from build123d import *

# Parameters (mm, degrees)
BASE_FLANGE1_DEPTH      = 70
CUT_EXTRUDE1_DEPTH      = 152.657508881
CUT_EXTRUDE1_DEPTH_BACK = 152.657508881
FILLET1_R               = 12
SKETCH7_R               = 4
SKETCH7_R_2             = 6
SKETCH7_R_3             = 7
CUT_EXTRUDE2_DEPTH      = 150.457314712
SKETCH8_R               = 5
CUT_EXTRUDE3_DEPTH      = 10
FILLET2_R               = 3
BOSS_EXTRUDE1_START     = 5
SKETCH9_R               = 10
SKETCH9_R_2             = 7
BOSS_EXTRUDE1_DEPTH     = 5
FILLET3_R               = 5
FILLET4_R               = 3
FILLET5_R               = 3
FILLET6_R               = 5
FILLET7_R               = 5


# Sheet-metal steps are written as plain solids
with BuildPart() as part:
    # Sketch1 → Base-Flange1 (new, symmetric)
    with BuildSketch(Plane(origin=(0, 0, 0), x_dir=(0, 0, -1), z_dir=(1, 0, 0))):
        with BuildLine():
            Line((-45, 100), (-45, 6))
            ThreePointArc((-45, 6), (-43.242640687, 1.757359313), (-39, 0))
            Line((-39, 0), (39, 0))
            ThreePointArc((39, 0), (43.242640687, 1.757359313), (45, 6))
            Line((45, 6), (45, 100))
            Line((45, 100), (42, 100))
            Line((42, 100), (42, 6))
            ThreePointArc((42, 6), (41.121320344, 3.878679656), (39, 3))
            Line((39, 3), (-39, 3))
            ThreePointArc((-39, 3), (-41.121320344, 3.878679656), (-42, 6))
            Line((-42, 6), (-42, 100))
            Line((-42, 100), (-45, 100))
        make_face()
    extrude(amount=BASE_FLANGE1_DEPTH, both=True)

    # Sketch6 → Cut-Extrude1 (cut, two sides: drawn at the far end of the back side and taken through both)
    with BuildSketch(Plane.XY.offset(45).offset(-CUT_EXTRUDE1_DEPTH_BACK)):
        Polygon((-417.259543972, 6), (-70, 6), (-60, 6), (-60, 70), (60, 100), (60, 6), (70, 6), (417.259543972, 6), (417.259543972, 700.519087943), (-417.259543972, 700.519087943), align=None)
    extrude(amount=CUT_EXTRUDE1_DEPTH + CUT_EXTRUDE1_DEPTH_BACK, mode=Mode.SUBTRACT)

    # Fillet1
    fillet1_edges = [part.edges().sort_by_distance(p)[0] for p in [
        (60, 100, -43.5),
        (60, 100, 43.5),
        (-60, 70, -43.5),
        (-60, 70, 43.5),
    ]]
    fillet(fillet1_edges, radius=FILLET1_R)

    # Sketch7 → Cut-Extrude2 (cut, through all)
    with BuildSketch(Plane.XY.offset(45)):
        with Locations((-48, 60.630683123)):
            Circle(SKETCH7_R)
        with Locations((48, 84.630683123)):
            Circle(SKETCH7_R_2)
        with Locations((-23, 38)):
            Circle(SKETCH7_R_3)
    extrude(amount=-CUT_EXTRUDE2_DEPTH, mode=Mode.SUBTRACT)

    # Sketch8 → Cut-Extrude3 (cut)
    with BuildSketch(Plane.XZ):
        with Locations(Location((7, 0, 0), (0, 0, 270))):
            Circle(SKETCH8_R)
        with Locations(Location((-50, 0, 0), (0, 0, 270))):
            Circle(SKETCH8_R)
        with BuildLine():
            Line((26, 5), (50, 5))
            ThreePointArc((50, 5), (55, 0), (50, -5))
            Line((50, -5), (26, -5))
            ThreePointArc((26, -5), (21, 0), (26, 5))
        make_face()
        with BuildLine():
            Line((-45, 27.5), (-45, 22.5))
            ThreePointArc((-45, 22.5), (-50, 17.5), (-55, 22.5))
            Line((-55, 22.5), (-55, 27.5))
            ThreePointArc((-55, 27.5), (-50, 32.5), (-45, 27.5))
        make_face()
        with BuildLine():
            Line((-45, -22.5), (-45, -27.5))
            ThreePointArc((-45, -27.5), (-50, -32.5), (-55, -27.5))
            Line((-55, -27.5), (-55, -22.5))
            ThreePointArc((-55, -22.5), (-50, -17.5), (-45, -22.5))
        make_face()
    extrude(amount=-CUT_EXTRUDE3_DEPTH, mode=Mode.SUBTRACT)

    # Fillet2
    fillet2_edges = [part.edges().sort_by_distance(p)[0] for p in [
        (-70, 6, -43.5),
        (70, 6, -43.5),
        (-70, 6, 43.5),
        (70, 6, 43.5),
    ]]
    fillet(fillet2_edges, radius=FILLET2_R - 0.0001)  # a hair under: the kernel refuses the full size

    # Sketch9 → Boss-Extrude1 (add)
    with BuildSketch(Plane.XY.offset(45).offset(BOSS_EXTRUDE1_START)):
        with Locations(Location((-23, 38, 0), (0, 0, 180))):
            Circle(SKETCH9_R)
        with Locations((-23, 38)):
            Circle(SKETCH9_R_2, mode=Mode.SUBTRACT)
    boss_extrude1 = extrude(amount=-BOSS_EXTRUDE1_DEPTH)

    # Fillet3
    fillet3_edges = [part.edges().sort_by_distance(p)[0] for p in [
        (-13, 38, 45),
    ]]
    fillet(fillet3_edges, radius=FILLET3_R - 0.0001)  # a hair under: the kernel refuses the full size

    # Fillet4
    fillet4_edges = [part.edges().sort_by_distance(p)[0] for p in [
        (-30, 38, 42),
    ]]
    fillet(fillet4_edges, radius=FILLET4_R)

    # Mirror5: Boss-Extrude1 across plane
    add(boss_extrude1.mirror(Plane.XY))

    # Fillet5
    fillet5_edges = [part.edges().sort_by_distance(p)[0] for p in [
        (-30, 38, -42),
    ]]
    fillet(fillet5_edges, radius=FILLET5_R)

    # Fillet6
    fillet6_edges = [part.edges().sort_by_distance(p)[0] for p in [
        (-13, 38, -45),
    ]]
    fillet(fillet6_edges, radius=FILLET6_R - 0.0001)  # a hair under: the kernel refuses the full size

    # Fillet7
    fillet7_edges = [part.edges().sort_by_distance(p)[0] for p in [
        (60, 6, -43.5),
        (60, 6, 43.5),
        (-60, 6, -43.5),
        (-60, 6, 43.5),
    ]]
    fillet(fillet7_edges, radius=FILLET7_R)


solid = part.part
CAD build for the part. Positions are in the model's coordinates, mm. A direction names the side the tool comes from. Give positions to 0.01 mm unless a question says otherwise; leave off trailing zeros. Write each loop counter-clockwise with the first axis right and the second up, starting at its lowest first coordinate (ties: lowest second). Pieces come first, ordered by that corner, then holes. Notation, with made-up numbers: (25.25, 38) -> (40.25, 38) arc R32 cw to (40.25, 75) -> close; hole circle Ø10 at (59, 7.25). An arc over 180 degrees is marked (long way). Return JSON: item names as keys, results as strings.
Item 1: Band-saw the part on D-D (y = 17). List the corners of the cut face in (x, z).
Answer below:
{"outline": "(-60, -45) -> (60, -45) -> (60, -42) -> (-60, -42) -> close; (-60, 42) -> (60, 42) -> (60, 45) -> (-60, 45) -> close"}
Item 2: Two-plate mould, pull along X, no slides. Class faces 6 (the cylindrical face through (43.58, 88.69, 43.52)), 7 (the flat face through (60, 48, 43)), 8 (the cylindrical face through (43.58, 88.69, -43.48)), 9 (the cylindrical face through (0.98, 1.711, -43.196)): +X half, -X half, draft (parallel to the pull), parting line (faces both ways), or undercut.
Answer below:
{"face 6": "undercut", "face 7": "+X half", "face 8": "undercut", "face 9": "draft"}
Item 3: Drill centre lines: probe 1 along X at (y, z) = (2, 0); probe 2 along Z at (x, y) = (-46, 17); probe 3 along Y at (x, z) = (28.5, 10.5). Where is each one in solid material? Low to high.
Answer below:
{"probe 1": "x = -70 to -55, -45 to 2, 12 to 21, 55 to 70", "probe 2": "z = -45 to -42, 42 to 45", "probe 3": "y = 0 to 3"}
Item 4: Band-saw the part on C-C (x = -3). List the corners of the cut face in (y, z).
Answer below:
{"outline": "(0, -39) arc R6 ccw to (6, -45) -> (84.25, -45) -> (84.25, -42) -> (6, -42) arc R3 cw to (3, -39) -> (3, 39) arc R3 cw to (6, 42) -> (84.25, 42) -> (84.25, 45) -> (6, 45) arc R6 ccw to (0, 39) -> close"}
Item 5: Drop flat-ended pins along their axis: pin 1 (15.5 mm diameter, centred on x = 48, y = 84.63, fed in from +Z); pin 2 (12 mm diameter, centred on x = 48.5, y = 13.5, fed in from -Z); pin 3 (8 mm diameter, centred on y = 83, z = 39, fed in from +X); pin 4 (9 mm diameter, centred on x = -50, z = 0, fed in from -Y). Give the stop position or say it passes through.
Answer below:
{"pin 1": "stops at z = 45", "pin 2": "stops at z = -45", "pin 3": "stops at x = 60", "pin 4": "passes through"}
Item 6: Tool access for faces 1 (the flat face through (1, 41, 42)), 2 (the cylindrical face through (-61, 8, -43)), 3 (the cylindrical face through (-48.5, 64.6, 43.5)), 4 (the cylindrical face through (55, 1, 0)), 5 (the flat face through (60, 48, -44)): list every direction of +Z, -Z, +X, -X, +Y, -Y with a clear straight run to the whole face (end or side of a thin tool).
Answer below:
{"face 1": "+X, -X, +Y", "face 2": "+Z, -Z, -X, +Y", "face 3": "+Z, -Z", "face 4": "+Y, -Y", "face 5": "+Z, -Z, +X, +Y"}
Item 7: Band-saw the part on B-B (y = 75). List the corners of the cut face in (x, z), then the cut area to 3 significant figures.
Answer below:
{"outline": "(-40, -45) -> (60, -45) -> (60, -42) -> (-40, -42) -> close; (-40, 42) -> (60, 42) -> (60, 45) -> (-40, 45) -> close", "area": "600 mm2"}
Item 8: Band-saw the part on A-A (x = 48). List the corners of the cut face in (y, z).
Answer below:
{"outline": "(0, -39) arc R6 ccw to (6, -45) -> (78.63, -45) -> (78.63, -42) -> (6, -42) arc R3 cw to (3, -39) -> (3, -5) -> (0, -5) -> close; (0, 5) -> (3, 5) -> (3, 39) arc R3 cw to (6, 42) -> (78.63, 42) -> (78.63, 45) -> (6, 45) arc R6 ccw to (0, 39) -> close; (90.63, -45) -> (96.63, -45) -> (96.63, -42) -> (90.63, -42) -> close; (90.63, 42) -> (96.63, 42) -> (96.63, 45) -> (90.63, 45) -> close"}
